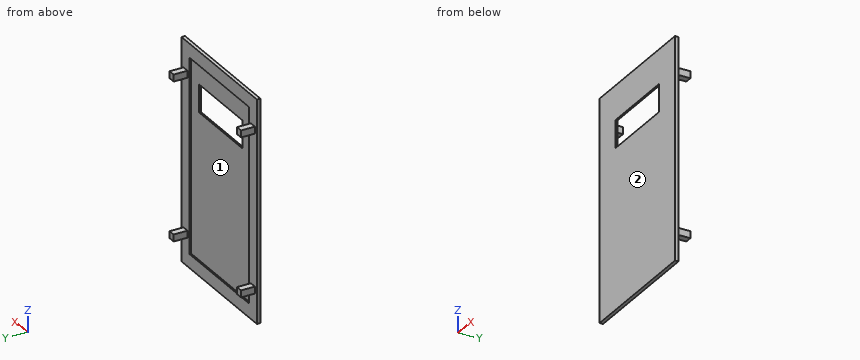
from build123d import *

# Parameters (mm, degrees)
SKETCH1_W           = 47
SKETCH1_H           = 80
BOSS_EXTRUDE1_DEPTH = 1.25
SKETCH2_W           = 2.5
SKETCH2_H           = 2.5
BOSS_EXTRUDE2_DEPTH = 5
SKETCH3_W           = 27
SKETCH3_H           = 10
CUT_EXTRUDE1_DEPTH  = 5
SKETCH6_W           = 37
SKETCH6_H           = 70
CUT_EXTRUDE2_DEPTH  = 0.6


with BuildPart() as part:
    # Sketch1 → Boss-Extrude1 (new body)
    with BuildSketch(Plane(origin=(0, 0, 0), x_dir=(1, 0, 0), z_dir=(0, 1, 0))):
        with Locations((23.5, 40)):
            Rectangle(SKETCH1_W, SKETCH1_H)
    extrude(amount=BOSS_EXTRUDE1_DEPTH)

    # Sketch2 → Boss-Extrude2 (add)
    with BuildSketch(Plane(origin=(0, 1.25, 0), x_dir=(1, 0, 0), z_dir=(0, 1, 0))):
        with Locations((44.5, 68.5)):
            Rectangle(SKETCH2_W, SKETCH2_H)
        with Locations((44.5, 11.5)):
            Rectangle(SKETCH2_W, SKETCH2_H)
        with Locations((2.5, 11.5)):
            Rectangle(SKETCH2_W, SKETCH2_H)
        with Locations((2.5, 68.5)):
            Rectangle(SKETCH2_W, SKETCH2_H)
    extrude(amount=BOSS_EXTRUDE2_DEPTH)

    # Sketch3 → Cut-Extrude1 (cut)
    with BuildSketch(Plane(origin=(0, 1.25, 0), x_dir=(1, 0, 0), z_dir=(0, 1, 0))):
        with Locations((23.5, 17.35)):
            Rectangle(SKETCH3_W, SKETCH3_H)
    extrude(amount=-CUT_EXTRUDE1_DEPTH, mode=Mode.SUBTRACT)

    # Sketch6 → Cut-Extrude2 (cut)
    with BuildSketch(Plane(origin=(0, 1.25, 0), x_dir=(1, 0, 0), z_dir=(0, 1, 0))):
        with Locations((23.5, 40)):
            Rectangle(SKETCH6_W, SKETCH6_H)
    extrude(amount=-CUT_EXTRUDE2_DEPTH, mode=Mode.SUBTRACT)


solid = part.part
Can you work these out from the model? Positions are in its coordinate system, mm. Face numbers are marked on the shaded views. Give positions to 0.01 mm unless a question says otherwise; leave off trailing zeros. Order: outer loops, then holes, each group sorted by start corner. A loop starts at its lowest first (then second) coordinate and runs counter-clockwise, first axis right, second up. Notation, with made-up numbers: (-10.75, 89.5) - (20.25, 89.5) arc R20 ccw to (20.25, 107.5) - close; hole circle Ø3 at (61.5, 82.5). An arc over 180 degrees is marked (long way). Write each question's results on one line, items separated by ' | '.
1) If we mould it in two halves opening along X, with no side actions, what happens to the marked faces 1 and 2? For each: pulls with the +X half, pulls with the -X half, needs draft (parallel to the pull), parting line crosses it, or undercut.
Final values:
face 1: undercut | face 2: needs draft
2) Please list where these lines run through material, in increasing order: line 1 along Z through (x, y) = (44, 1.75); line 2 along Y through (x, z) = (35.5, -36.5); line 3 along Y through (x, z) = (43, -69.5). Write a range as [from, to].
Final values:
line 1: z = [-69.75, -67.25], [-12.75, -10.25] | line 2: y = [0, 0.65] | line 3: y = [0, 1.25]
3) Suppose I cut it at B-B, the plane x = 27. Write out the boundary of the cut face in (y, z).
Final values:
outline: (0, -80) - (1.25, -80) - (1.25, -75) - (0.65, -75) - (0.65, -22.35) - (0, -22.35) - close; (0, -12.35) - (0.65, -12.35) - (0.65, -5) - (1.25, -5) - (1.25, 0) - (0, 0) - close
4) Suppose I cut it at D-D, the plane x = 3. Write out the boundary of the cut face in (y, z), then the cut area to 3 significant figures.
Final values:
outline: (0, -80) - (1.25, -80) - (1.25, -69.75) - (6.25, -69.75) - (6.25, -67.25) - (1.25, -67.25) - (1.25, -12.75) - (6.25, -12.75) - (6.25, -10.25) - (1.25, -10.25) - (1.25, 0) - (0, 0) - close | area: 125 mm^2
5) I'm going to push flat-ended pins straight in: pin 1 Ø18.5 at (x, z) = (20.5, -54) entering from +Y; pin 2 Ø2 at (x, y) = (45, 3) entering from +Z; pin 3 Ø0.8 at (x, y) = (44, 3.5) entering from -Z. Where does each tip first touch, or does it pass through?
Final values:
pin 1: stops at y = 0.65 | pin 2: stops at z = -10.25 | pin 3: stops at z = -69.75
6) Suppose I cut it at A-A, the plane y = 3. Write out the boundary of the cut face in (x, z).
Final values:
outline: (1.25, -69.75) - (3.75, -69.75) - (3.75, -67.25) - (1.25, -67.25) - close; (1.25, -12.75) - (3.75, -12.75) - (3.75, -10.25) - (1.25, -10.25) - close; (43.25, -69.75) - (45.75, -69.75) - (45.75, -67.25) - (43.25, -67.25) - close; (43.25, -12.75) - (45.75, -12.75) - (45.75, -10.25) - (43.25, -10.25) - close
7) Suppose I cut it at C-C, the plane z = -30. Write out the boundary of the cut face in (x, y), then the cut area to 4 significant figures.
Final values:
outline: (0, 0) - (47, 0) - (47, 1.25) - (42, 1.25) - (42, 0.65) - (5, 0.65) - (5, 1.25) - (0, 1.25) - close | area: 36.55 mm^2
